Check sheet for the modelled part. Datum: model origin and axes. Units: mm. Face numbers are marked on the shaded views. A direction names the side the tool comes from. Round coordinates to 2 decimals unless told otherwise and drop trailing zeros. Loops run counter-clockwise (first coordinate to the right, second up) from the corner with the lowest first, then second, coordinate; pieces in that order, holes last. Notation, with made-up numbers: (-24, 4) -> (34, 4) arc R13 cw to (34, 19) -> close; hole circle Ø5 at (13.5, 56.5). An arc over 180 degrees is marked (long way). Return JSON: item names as keys, results as strings.
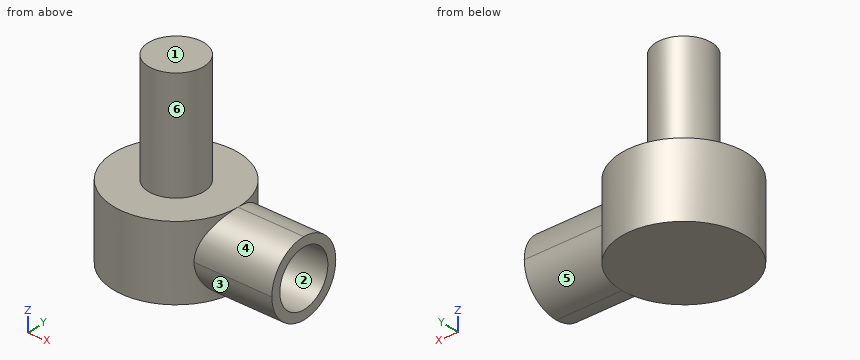
from build123d import *

# Parameters (mm, degrees)
BOSS_EXTRUDE1_DEPTH = 40
SKETCH2_R           = 15.05
CUT_EXTRUDE1_DEPTH  = 40
FILLET1_R           = 20
SKETCH3_R           = 15
BOSS_EXTRUDE2_DEPTH = 60


with BuildPart() as part:
    # Sketch1 → Boss-Extrude1 (new body)
    with BuildSketch(Plane.XY):
        with BuildLine():
            Line((27.270825141, -20), (70, -20))
            Line((70, -20), (70, 20))
            Line((70, 20), (27.270825141, 20))
            ThreePointArc((27.270825141, 20), (-33.818602926, 0), (27.270825141, -20))
        make_face()
    extrude(amount=BOSS_EXTRUDE1_DEPTH)

    # Sketch2 → Cut-Extrude1 (cut)
    with BuildSketch(Plane(origin=(70, 0, 0), x_dir=(0, 0, -1), z_dir=(1, 0, 0))):
        with Locations((-20, 0)):
            Circle(SKETCH2_R)
    extrude(amount=-CUT_EXTRUDE1_DEPTH, mode=Mode.SUBTRACT)

    # Fillet1
    fillet1_edges = [part.edges().sort_by_distance(p)[0] for p in [
        (48.635412571, 20, 40),
        (48.635412571, -20, 40),
        (48.635412571, -20, 0),
        (48.635412571, 20, 0),
    ]]
    fillet(fillet1_edges, radius=FILLET1_R - 0.0001)  # a hair under: the kernel refuses the full size

    # Sketch3 → Boss-Extrude2 (add)
    with BuildSketch(Plane.XY.offset(40)):
        Circle(SKETCH3_R)
    extrude(amount=BOSS_EXTRUDE2_DEPTH)


solid = part.part
Q1. Section check C-C (y = 5). Record the boundary of the cut face in (x, z).
Results list:
{"outline": "(-33.45, 0) -> (33.45, 0) -> (33.45, 0.64) -> (70, 0.64) -> (70, 5.8) -> (30, 5.8) -> (30, 34.2) -> (70, 34.2) -> (70, 39.36) -> (33.45, 39.36) -> (33.45, 40) -> (14.14, 40) -> (14.14, 100) -> (-14.14, 100) -> (-14.14, 40) -> (-33.45, 40) -> close"}
Q2. Draft check along Z on the marked faces 1, 2 and 3. Enter one of: released by +Z, released by -Z, zero draft, split by the parting line, or undercut.
Results list:
{"face 1": "released by +Z", "face 2": "undercut", "face 3": "released by -Z"}
Q3. Section check D-D (z = 6.5). Record the boundary of the cut face in (x, y), then the cut area to 3 significant figures.
Results list:
{"outline": "(30, -6.65) -> (30, 6.65) -> (70, 6.65) -> (70, 14.76) -> (30.43, 14.76) arc R33.82 ccw (long way) to (30.43, -14.76) -> (70, -14.76) -> (70, -6.65) -> close", "area": "4,160 mm^2"}
Q4. Section check B-B (x = 0). Record the boundary of the cut face in (y, z), then the cut area to 3 significant figures.
Results list:
{"outline": "(-33.82, 0) -> (33.82, 0) -> (33.82, 40) -> (15, 40) -> (15, 100) -> (-15, 100) -> (-15, 40) -> (-33.82, 40) -> close", "area": "4,510 mm^2"}
Q5. Tool access check on the marked faces 4, 5 and 6. Record the directions out of +Z, -Z, +X, -X, +Y, -Y that give a thin tool (end or side, any length) a straight path to the whole face; none if there is none.
Results list:
{"face 4": "+Z, +X, -Y", "face 5": "-Z, +X, +Y", "face 6": "+Z"}
Q6. Go/stop test with flat-tipped pins: pin 1 (4 mm diameter, centred on y = -21.5, z = 35.5, fed in from +X); pin 2 (1.5 mm diameter, centred on x = 44, y = 22.5, fed in from -Z); pin 3 (12 mm diameter, centred on x = 18.5, y = -24.5, fed in from +Z); pin 4 (5 mm diameter, centred on x = 6, z = 87.5, fed in from +Y). Record where each tip stops, or that it passes through.
Results list:
{"pin 1": "x = 27.63", "pin 2": "through", "pin 3": "z = 40", "pin 4": "y = 14.59"}
Q7. Material ranges on line 1 (Y direction, x = 62, z = 20); line 2 (Z direction, x = -4, y = 19); line 3 (X direction, y = 0.5, z = 17), recorded low to high.
Results list:
{"line 1": "-20 to -15.05, 15.05 to 20", "line 2": "0 to 40", "line 3": "-33.81 to 30"}
